Work out the finished part from the listing and answer in its coordinate system (mm). Face numbers are marked on the shaded views. A direction names the side the tool comes from. Round coordinates to 2 decimals unless told otherwise and drop trailing zeros. Order: outer loops, then holes, each group sorted by start corner. A loop starts at its lowest first (then second) coordinate and runs counter-clockwise, first axis right, second up. Notation, with made-up numbers: M 22.5,60.25 L 49.5,60.25 A33 ccw 49.5,92.25 Z; hole C 10.25,-7 d6. An arc over 180 degrees is marked long. Return JSON: item names as keys, results as strings.
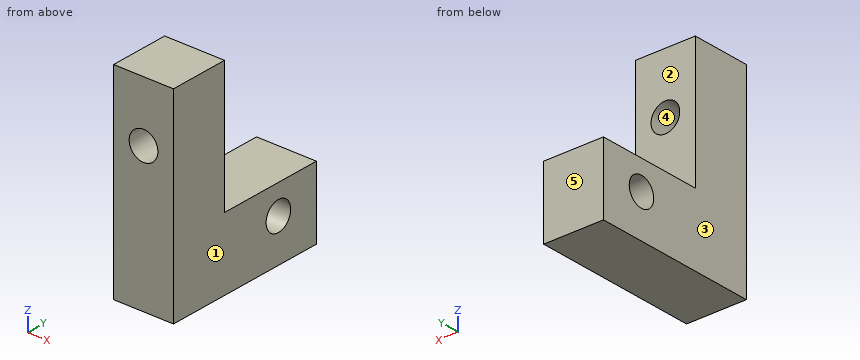
from build123d import *

# Parameters (mm, degrees)
BOSS_EXTRUDE1_DEPTH = 6.35
SKETCH4_R           = 1.524
CUT_EXTRUDE1_DEPTH  = 6.35
SKETCH5_R           = 1.524
CUT_EXTRUDE3_DEPTH  = 7.35


with BuildPart() as part:
    # Sketch3 → Boss-Extrude1 (new body)
    with BuildSketch(Plane(origin=(0, 0, 0), x_dir=(0, 0, -1), z_dir=(1, 0, 0))):
        Polygon((0, 0), (0, 6.35), (13.97, 6.35), (13.97, 17.78), (21.59, 17.78), (21.59, 0), align=None)
    extrude(amount=BOSS_EXTRUDE1_DEPTH)

    # Sketch4 → Cut-Extrude1 (cut)
    with BuildSketch(Plane(origin=(0, 6.35, 0), x_dir=(1, 0, 0), z_dir=(0, 1, 0))):
        with Locations((3.175, 6.35)):
            Circle(SKETCH4_R)
    extrude(amount=-CUT_EXTRUDE1_DEPTH, mode=Mode.SUBTRACT)

    # Sketch5 → Cut-Extrude3 (cut, through all)
    with BuildSketch(Plane(origin=(6.35, 0, 0), x_dir=(0, 0, -1), z_dir=(1, 0, 0))):
        with Locations((17.057623492, 13.051566734)):
            Circle(SKETCH5_R)
    extrude(amount=-CUT_EXTRUDE3_DEPTH, mode=Mode.SUBTRACT)


solid = part.part
Item 1: Find section B-B (z = -6.35). Determine the outline of the cut face in (x, y), plus the area to 3 significant figures.
Output:
{"outline": "M 0,0 L 1.65,0 L 1.65,6.35 L 0,6.35 Z; M 4.7,0 L 6.35,0 L 6.35,6.35 L 4.7,6.35 Z", "area": "21.0 mm^2"}
Item 2: Find section A-A (x = 2.25). Determine the outline of the cut face in (y, z), plus the area to 3 significant figures.
Output:
{"outline": "M 0,-21.59 L 17.78,-21.59 L 17.78,-13.97 L 6.35,-13.97 L 6.35,-7.56 L 0,-7.56 Z; M 0,-5.14 L 6.35,-5.14 L 6.35,0 L 0,0 Z; hole C 13.05,-17.06 d3.05", "area": "202 mm^2"}
Item 3: Consider line 1 along X through (y, z) = (4.25, -6.35); line 2 along Z through (x, y) = (6.25, 13); line 3 along Y through (x, z) = (2, -13). Determine where each line is inside the solid, lowest interval first. Write a range as [from, to].
Output:
{"line 1": "x = [0, 1.65], [4.7, 6.35]", "line 2": "z = [-21.59, -18.58], [-15.53, -13.97]", "line 3": "y = [0, 6.35]"}
Item 4: Find section D-D (x = 5.5). Determine the outline of the cut face in (y, z), plus the area to 3 significant figures.
Output:
{"outline": "M 0,-21.59 L 17.78,-21.59 L 17.78,-13.97 L 6.35,-13.97 L 6.35,0 L 0,0 Z; hole C 13.05,-17.06 d3.05", "area": "217 mm^2"}
Item 5: Which of the six approach directions +Z, -Z, +X, -X, +Y, -Y give full straight-line access (tool end or side, diameter ignored) to the marked faces 1 and 2?
Output:
{"face 1": "+Z, -Z, +X, +Y, -Y", "face 2": "+Z, +X, -X, +Y"}
Item 6: Find section C-C (y = 13.75). Determine the outline of the cut face in (x, z), plus the area to 3 significant figures.
Output:
{"outline": "M 0,-21.59 L 6.35,-21.59 L 6.35,-18.41 L 0,-18.41 Z; M 0,-15.7 L 6.35,-15.7 L 6.35,-13.97 L 0,-13.97 Z", "area": "31.2 mm^2"}
Item 7: Each of these flat-tipped pins is pushed along its axis until it touches: pin 1 (1.9 mm diameter, centred on x = 3, y = 13, fed in from +Z); pin 2 (3 mm diameter, centred on x = 3, z = -6.5, fed in from +Y). Where does it stop, or does it pass through?
Output:
{"pin 1": "stops at z = -13.97", "pin 2": "stops at y = 6.35"}
Item 8: The mould has two halves that part along X. Classify the marked faces 3, 4 and 5: pulls with the +X half, pulls with the -X half, needs draft (parallel to the pull), parting line crosses it, or undercut.
Output:
{"face 3": "pulls with the -X half", "face 4": "undercut", "face 5": "needs draft"}
